Verification items for the finished model (mm, model axes). Face numbers are marked on the shaded views. A direction names the side the tool comes from. Round coordinates to 2 decimals unless told otherwise and drop trailing zeros. Write each loop counter-clockwise with the first axis right and the second up, starting at its lowest first coordinate (ties: lowest second). Pieces come first, ordered by that corner, then holes. Notation, with made-up numbers: M 44,-33.5 L 96,-33.5 A15 ccw 96,-29.5 Z; hole C 5,45.5 d9. An arc over 180 degrees is marked long. One line per question, with ' | ' between items.
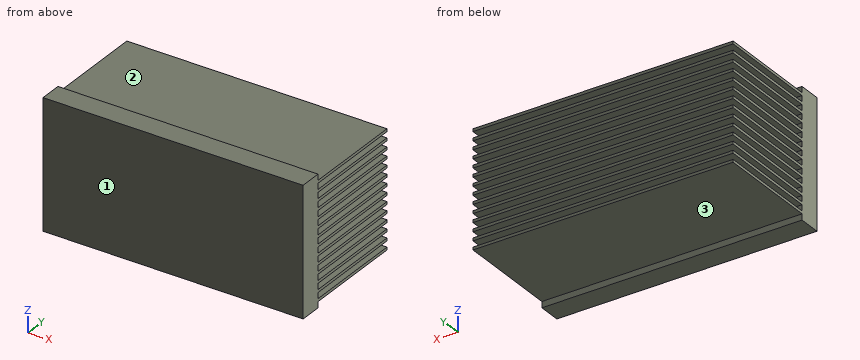
from build123d import *

# Parameters (mm, degrees)
SKETCH1_W           = 152
SKETCH1_H           = 75
BOSS_EXTRUDE1_DEPTH = 73
SKETCH2_W           = 152
SKETCH2_H           = 3.5
CUT_EXTRUDE1_DEPTH  = 60


with BuildPart() as part:
    # Sketch1 → Boss-Extrude1 (new body)
    with BuildSketch(Plane(origin=(0, 0, 0), x_dir=(1, 0, 0), z_dir=(0, 1, 0))):
        with Locations((76, 37.5)):
            Rectangle(SKETCH1_W, SKETCH1_H)
    extrude(amount=BOSS_EXTRUDE1_DEPTH)

    # Sketch2 → Cut-Extrude1 (cut)
    with BuildSketch(Plane(origin=(0, 73, 0), x_dir=(1, 0, 0), z_dir=(0, 1, 0))):
        with Locations((76, 1.75)):
            Rectangle(SKETCH2_W, SKETCH2_H)
        with Locations((76, 6.857142857)):
            Rectangle(SKETCH2_W, SKETCH2_H)
        with Locations((76, 11.964285714)):
            Rectangle(SKETCH2_W, SKETCH2_H)
        with Locations((76, 17.071428571)):
            Rectangle(SKETCH2_W, SKETCH2_H)
        with Locations((76, 22.178571429)):
            Rectangle(SKETCH2_W, SKETCH2_H)
        with Locations((76, 27.285714286)):
            Rectangle(SKETCH2_W, SKETCH2_H)
        with Locations((76, 32.392857143)):
            Rectangle(SKETCH2_W, SKETCH2_H)
        with Locations((76, 37.5)):
            Rectangle(SKETCH2_W, SKETCH2_H)
        with Locations((76, 42.607142857)):
            Rectangle(SKETCH2_W, SKETCH2_H)
        with Locations((76, 47.714285714)):
            Rectangle(SKETCH2_W, SKETCH2_H)
        with Locations((76, 52.821428571)):
            Rectangle(SKETCH2_W, SKETCH2_H)
        with Locations((76, 57.928571429)):
            Rectangle(SKETCH2_W, SKETCH2_H)
        with Locations((76, 63.035714286)):
            Rectangle(SKETCH2_W, SKETCH2_H)
        with Locations((76, 68.142857143)):
            Rectangle(SKETCH2_W, SKETCH2_H)
        with Locations((76, 73.25)):
            Rectangle(SKETCH2_W, SKETCH2_H)
    extrude(amount=-CUT_EXTRUDE1_DEPTH, mode=Mode.SUBTRACT)


solid = part.part
1. Section check A-A, the plane y = 32. Count the separate pieces of the cut face and the enclosed holes in it, then the cut area to 3 significant figures.
Results:
separate pieces: 14 | enclosed holes: 0 | area: 3,420 mm2
2. Tool access check on the marked faces 1, 2 and 3. Record the directions out of +Z, -Z, +X, -X, +Y, -Y that give a thin tool (end or side, any length) a straight path to the whole face; none if there is none.
Results:
face 1: +Z, -Z, +X, -X, -Y | face 2: +Z, +X, -X, +Y | face 3: -Z, +X, -X, +Y
3. Go/stop test with flat-tipped pins: P1, Ø1.8, axis at x = 44.5, z = -42, coming from the +Y side; P2, Ø4, axis at x = 112.5, z = -32.5, coming from the +Y side; P3, Ø18, axis at x = 46.5, y = 35, coming from the +Z side; P4, Ø1, axis at y = 60.5, z = -16, coming from the -X side. Record where each tip stops, or that it passes through.
Results:
P1: stops at y = 13 | P2: stops at y = 73 | P3: stops at z = -3.5 | P4: passes through
4. Thickness scan on line 1 (Y direction, x = 100, z = -16.5). Record the ranges inside material, lowest first.
Results:
line 1: y = 0 to 13
5. Section check B-B, the plane z = -17. Record the cut outline in (x, y), then the cut area to 3 significant figures.
Results:
outline: M 0,0 L 152,0 L 152,13 L 0,13 Z | area: 1,980 mm2
